Source: CAD feature listing. Evaluate the final solid. Frame: model axes, mm. Face numbers are marked on the shaded views. A direction names the side the tool comes from. Coordinates: 2 decimals unless noted, no trailing zeros. Loops run counter-clockwise (first coordinate to the right, second up) from the corner with the lowest first, then second, coordinate; pieces in that order, holes last. Notation, with made-up numbers: (-30, 53.25) - (19, 53.25) arc R20 ccw to (19, 72.25) - close; hole circle Ø7 at (56, 59.25). An arc over 180 degrees is marked (long way). Write item = value, one per line. Start each with the question number.
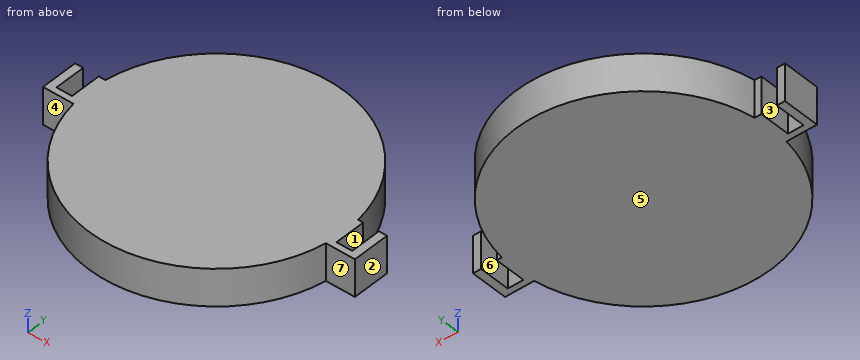
from build123d import *

# Parameters (mm, degrees)
F1_DEPTH = 2.54


with BuildPart() as f1:
    # F0 (on Top) → F1 (new body)
    with BuildSketch(Plane.XY):
        with BuildLine():
            ThreePointArc((8.6617718357, -1.3281105626), (8.7376563104, -0.6659813826), (8.763, 0))
            ThreePointArc((8.763, 0), (8.7419235528, 0.6074056285), (8.6787955957, 1.2118894374))
            Line((8.6787955957, 1.2118894374), (-8.6787955957, 1.2118894374))
            ThreePointArc((-8.6787955957, 1.2118894374), (-8.7628031879, -0.0587306529), (-8.6617718357, -1.3281105626))
            Line((-8.6617718357, -1.3281105626), (8.6617718357, -1.3281105626))
        make_face()
        with BuildLine():
            Line((-8.6787955957, 1.2118894374), (8.6787955957, 1.2118894374))
            ThreePointArc((8.6787955957, 1.2118894374), (0, 8.763), (-8.6787955957, 1.2118894374))
        make_face()
        with BuildLine():
            ThreePointArc((-8.6617718357, -1.3281105626), (0, -8.763), (8.6617718357, -1.3281105626))
            Line((8.6617718357, -1.3281105626), (-8.6617718357, -1.3281105626))
        make_face()
        with BuildLine():
            ThreePointArc((8.6787955957, 1.2118894374), (8.7419235528, 0.6074056285), (8.763, 0))
            ThreePointArc((8.763, 0), (8.7376563104, -0.6659813826), (8.6617718357, -1.3281105626))
            Line((8.6617718357, -1.3281105626), (10.6583032757, -1.3281105626))
            Line((10.6583032757, -1.3281105626), (10.6583032757, 1.2118894374))
            Line((10.6583032757, 1.2118894374), (10.1039223373, 1.2118894374))
            Line((10.1039223373, 1.2118894374), (10.1039223373, -0.9020056459))
            Line((10.1039223373, -0.9020056459), (9.0270256624, -0.9020056459))
            Line((9.0270256624, -0.9020056459), (9.0270256624, 1.2118894374))
            Line((9.0270256624, 1.2118894374), (8.6787955957, 1.2118894374))
        make_face()
        with BuildLine():
            ThreePointArc((-8.6617718357, -1.3281105626), (-8.7628031879, -0.0587306529), (-8.6787955957, 1.2118894374))
            Line((-8.6787955957, 1.2118894374), (-9.1322259977, 1.2118894374))
            Line((-9.1322259977, 1.2118894374), (-9.1322259977, 1.1553943541))
            Line((-9.1322259977, 1.1553943541), (-9.1322259977, -0.9020056459))
            Line((-9.1322259977, -0.9020056459), (-10.2012958378, -0.9020056459))
            Line((-10.2012958378, -0.9020056459), (-10.2012958378, 1.1553943541))
            Line((-10.2012958378, 1.1553943541), (-10.2012958378, 1.2118894374))
            Line((-10.2012958378, 1.2118894374), (-10.7550928369, 1.2118894374))
            Line((-10.7550928369, 1.2118894374), (-10.7550928369, -1.3281105626))
            Line((-10.7550928369, -1.3281105626), (-8.6617718357, -1.3281105626))
        make_face()
    extrude(amount=F1_DEPTH)


solid = f1.part
Item 1: Material intervals for L1, parallel to X at y = -0.5, z = 2.3; L2, parallel to Y at x = 8.75, z = 0.2; L3, parallel to Y at x = 9.5, z = 0.6, sorted ascending. Write a range as [from, to].
Item 2: Reachability of the marked faces 5, 6 and 7 from +Z, -Z, +X, -X, +Y, -Y: full face, straight path, thin tool, end or side. Return the list, or none.
Item 3: Cut plane C-C (y = -3.5). Return the cut outline in (x, z), then the cut area to 3 significant figures.
Item 4: Draft query along X for the marked faces 1, 2, 3 and 4. Return one class per face: released by +X, released by -X, zero draft, split by the parting line, or undercut.
Item 5: First-contact query: pin 1 (6 mm diameter, centred on x = 8.5, y = 4, fed in from +Z); pin 2 (0.5 mm diameter, centred on x = 9.5, z = 1.5, fed in from +Y). Flat tips, straight axial feed; report the tip coordinate or a pass-through.
Item 6: Cut plane B-B (x = 9.25). Return the cut outline in (y, z).
Item 7: Cut plane A-A (z = 1.7). Return the cut outline in (x, y).
Responses:
q1.L1 = [-10.76, -10.2], [-9.13, 9.03], [10.1, 10.66]
q1.L2 = [-1.33, 1.21]
q1.L3 = [-1.33, -0.9]
q2.face_5 = -Z, +X, -X, +Y, -Y
q2.face_6 = +Z, -Z, +Y
q2.face_7 = +Z, -Z, +X, -Y
q3.outline = (-8.03, 0) - (8.03, 0) - (8.03, 2.54) - (-8.03, 2.54) - close
q3.area = 40.8 mm2
q4.face_1 = undercut
q4.face_2 = released by +X
q4.face_3 = undercut
q4.face_4 = zero draft
q5.pin_1 = 2.54
q5.pin_2 = -0.9
q6.outline = (-1.33, 0) - (-0.9, 0) - (-0.9, 2.54) - (-1.33, 2.54) - close
q7.outline = (-10.76, -1.33) - (-8.66, -1.33) arc R8.76 ccw to (8.66, -1.33) - (10.66, -1.33) - (10.66, 1.21) - (10.1, 1.21) - (10.1, -0.9) - (9.03, -0.9) - (9.03, 1.21) - (8.68, 1.21) arc R8.76 ccw to (-8.68, 1.21) - (-9.13, 1.21) - (-9.13, -0.9) - (-10.2, -0.9) - (-10.2, 1.21) - (-10.76, 1.21) - close
